Verification items for this drawing (mm, ordinates from the low corner). Round coordinates to 2 decimals unless told otherwise and drop trailing zeros. Order: outer loops, then holes, each group sorted by start corner. A loop starts at its lowest first (then second) coordinate and runs counter-clockwise, first axis right, second up. Notation, with made-up numbers: (-35.75, -18.75) -> (4.25, -18.75) arc R21 cw to (4.25, 1.25) -> close; hole circle Ø2 at (26.5, 42.5). An arc over 180 degrees is marked (long way). Answer in a Markdown table with one row per item. Add a question column.
1. Depth check by flat-ended pin: P1, Ø2.5, axis at x = 61.5, z = 3.5, coming from the +Y side. Enter the tip coordinate at first touch or a pass-through.
2. Sectioned sample at A-A, the plane x = 54. Record the boundary of the cut face in (y, z).
3. Material ranges on L1, parallel to X at y = 0.5, z = 26.5; L2, parallel to X at y = 0.5, z = 3.5 (1 decimal); L3, parallel to Z at x = 54.5, y = 1.4, recorded low to high. Write a range as from..to.
4. Sectioned sample at B-B, the plane y = 0.55. Record the boundary of the cut face in (x, z) (1 decimal).
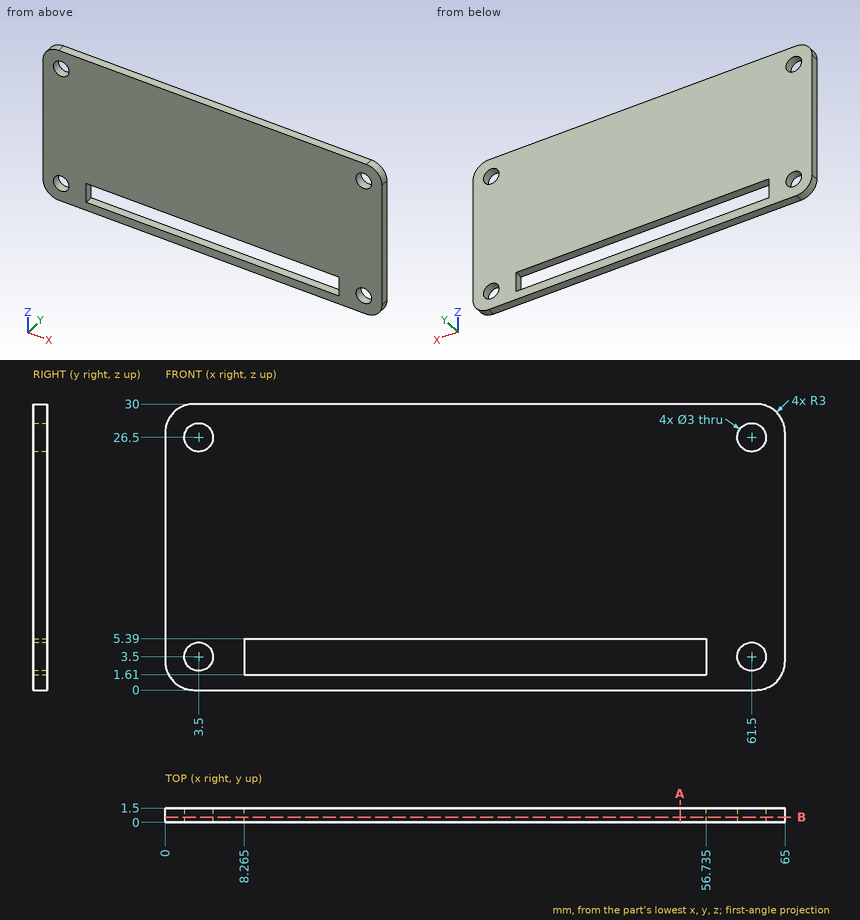
Answer key:
| question | item | result |
|---|---|---|
| 1 | P1 | passes through |
| 2 | outline | (0, 0) -> (1.5, 0) -> (1.5, 1.61) -> (0, 1.61) -> close; (0, 5.39) -> (1.5, 5.39) -> (1.5, 30) -> (0, 30) -> close |
| 3 | L1 | x = 0..2, 5..60, 63..65 |
| 3 | L2 | x = 0..2, 5..8.3, 56.7..60, 63..65 |
| 3 | L3 | z = 0..1.61, 5.39..30 |
| 4 | outline | (0, 3) arc R3 ccw to (3, 0) -> (62, 0) arc R3 ccw to (65, 3) -> (65, 27) arc R3 ccw to (62, 30) -> (3, 30) arc R3 ccw to (0, 27) -> close; hole circle Ø3 at (3.5, 3.5); hole circle Ø3 at (3.5, 26.5); hole (8.3, 1.6) -> (56.7, 1.6) -> (56.7, 5.4) -> (8.3, 5.4) -> close; hole circle Ø3 at (61.5, 3.5); hole circle Ø3 at (61.5, 26.5) |
